from build123d import *

# Parameters (mm, degrees)
BOSS_EXTRUDE1_DEPTH     = 8
SKETCH1_W               = 122.5
SKETCH1_H               = 80
BOSS_EXTRUDE1_2_DEPTH   = 8
BOSS_EXTRUDE2_DEPTH     = 53.5
CUT_EXTRUDE6_DEPTH      = 7.5
SKETCH2_W               = 60
SKETCH2_H               = 31
SKETCH2_R               = 2.25
BOSS_EXTRUDE3_DEPTH     = 31.5
CUT_EXTRUDE5_REACH      = 165.406
SKETCH8_W               = 15.75
SKETCH8_H               = 31
CUT_EXTRUDE8_START      = -3
CUT_EXTRUDE8_DEPTH      = 3
FILLET1_R               = 3
CUT_EXTRUDE1_DEPTH      = 122.5
CUT_EXTRUDE1_DEPTH_BACK = 15
SKETCH4_W               = 3
SKETCH4_H               = 87.5
BOSS_EXTRUDE5_DEPTH     = 122.5
SKETCH5_W               = 5
SKETCH5_H               = 80
CUT_EXTRUDE2_DEPTH      = 122.5
CUT_EXTRUDE3_DEPTH      = 15
CUT_EXTRUDE3_DEPTH_BACK = 92.5
SKETCH7_R               = 2.25
CUT_EXTRUDE4_DEPTH      = 13.5
CUT_EXTRUDE9_DEPTH      = 5
SKETCH13_R              = 1.75
CUT_EXTRUDE10_DEPTH     = 7.5


with BuildPart() as part:
    # Sketch1 → Boss-Extrude1 (new body)
    with BuildSketch(Plane.XY):
        Polygon((32.428932188, 92.5), (27.5, 92.5), (27.5, 7.5), (-92.5, 7.5), (-92.5, -92.5), (92.5, -92.5), (92.5, 32.428932188), align=None)
    extrude(amount=BOSS_EXTRUDE1_DEPTH)



with BuildPart() as body_2:
    # Sketch1 → Boss-Extrude1 2 (new body)
    with BuildSketch(Plane.XY):
        with Locations((-38.75, 52.5)):
            Rectangle(SKETCH1_W, SKETCH1_H)
    extrude(amount=BOSS_EXTRUDE1_2_DEPTH)


with BuildPart() as part_1:
    add(part.part)

    add(body_2.part)  # Boss-Extrude2 merges body 2
    # Sketch1<4> → Boss-Extrude2 (add)
    with BuildSketch(Plane.XY):
        Polygon((22.5, 92.5), (22.5, 12.5), (-100, 12.5), (-100, -100), (100, -100), (100, 32), (32, 100), (-100, 100), (-100, 92.5), align=None)
        Polygon((-92.5, 7.5), (27.5, 7.5), (27.5, 92.5), (32.428932188, 92.5), (92.5, 32.428932188), (92.5, -92.5), (-92.5, -92.5), align=None, mode=Mode.SUBTRACT)
    extrude(amount=BOSS_EXTRUDE2_DEPTH)

    # Sketch9 → Cut-Extrude6 (cut)
    with BuildSketch(Plane.XZ.offset(100)):
        with BuildLine():
            Line((-90, 42.466293919), (90, 42.466293919))
            ThreePointArc((90, 42.466293919), (94, 46.466293919), (90, 50.466293919))
            Line((90, 50.466293919), (-90, 50.466293919))
            ThreePointArc((-90, 50.466293919), (-94, 46.466293919), (-90, 42.466293919))
        make_face()
        with BuildLine():
            Line((-90, 26.466293919), (90, 26.466293919))
            ThreePointArc((90, 26.466293919), (94, 30.466293919), (90, 34.466293919))
            Line((90, 34.466293919), (-90, 34.466293919))
            ThreePointArc((-90, 34.466293919), (-94, 30.466293919), (-90, 26.466293919))
        make_face()
        with BuildLine():
            Line((-90, 10.466293919), (90, 10.466293919))
            ThreePointArc((90, 10.466293919), (94, 14.466293919), (90, 18.466293919))
            Line((90, 18.466293919), (-90, 18.466293919))
            ThreePointArc((-90, 18.466293919), (-94, 14.466293919), (-90, 10.466293919))
        make_face()
    extrude(amount=-CUT_EXTRUDE6_DEPTH, mode=Mode.SUBTRACT)

    # Sketch2 → Boss-Extrude3 (add)
    with BuildSketch(Plane.XY.offset(8)):
        with Locations((12.359091867, -30)):
            Rectangle(SKETCH2_W, SKETCH2_H)
        with BuildLine():
            ThreePointArc((-14.640908133, -38.997517342), (-11.721838066, -37.877814495), (-10.5, -35))
            Line((-10.5, -35), (-10.5, -25))
            ThreePointArc((-10.5, -25), (-11.721838066, -22.122185505), (-14.640908133, -21.002482658))
            Line((-14.640908133, -21.002482658), (-14.640908133, -17.5))
            Line((-14.640908133, -17.5), (34.640908133, -17.5))
            Line((34.640908133, -17.5), (34.640908133, -21.002482658))
            ThreePointArc((34.640908133, -21.002482658), (31.721838066, -22.122185505), (30.5, -25))
            Line((30.5, -25), (30.5, -35))
            ThreePointArc((30.5, -35), (31.721838066, -37.877814495), (34.640908133, -38.997517342))
            Line((34.640908133, -38.997517342), (34.640908133, -42.5))
            Line((34.640908133, -42.5), (-14.640908133, -42.5))
            Line((-14.640908133, -42.5), (-14.640908133, -38.997517342))
        make_face(mode=Mode.SUBTRACT)
        with Locations((-14.5, -25)):
            Circle(SKETCH2_R, mode=Mode.SUBTRACT)
        with Locations((-14.5, -35)):
            Circle(SKETCH2_R, mode=Mode.SUBTRACT)
        with Locations((34.5, -35)):
            Circle(SKETCH2_R, mode=Mode.SUBTRACT)
        with Locations((34.5, -25)):
            Circle(SKETCH2_R, mode=Mode.SUBTRACT)
    extrude(amount=BOSS_EXTRUDE3_DEPTH)

    # Cut-Extrude5: up to this face of the body (flat: up to its plane)
    cut_extrude5_end = Plane(part_1.part.faces().sort_by_distance((-10.5, -30, 23.75))[0])
    # Sketch8 → Cut-Extrude5 (cut, up to the picked face)
    with BuildSketch(Plane.ZY.offset(17.640908133), mode=Mode.PRIVATE) as cut_extrude5_sk1:
        with Locations((15.875, -30)):
            Rectangle(SKETCH8_W, SKETCH8_H)
    cut_extrude5_tool1 = split(extrude(cut_extrude5_sk1.sketch, amount=-CUT_EXTRUDE5_REACH, mode=Mode.PRIVATE), bisect_by=cut_extrude5_end, keep=Keep.BOTH, mode=Mode.PRIVATE)
    add(cut_extrude5_tool1.solids().sort_by(Axis((-17.640908, -30, 15.875), (1, 0, 0)))[0], mode=Mode.SUBTRACT)

    # Sketch10 → Cut-Extrude8 (cut)
    with BuildSketch(Plane.XY.offset(8).offset(CUT_EXTRUDE8_START)):
        with BuildLine():
            Line((34.640908133, -42.5), (34.640908133, -38.997517342))
            ThreePointArc((34.640908133, -38.997517342), (31.721838066, -37.877814495), (30.5, -35))
            Line((30.5, -35), (30.5, -25))
            ThreePointArc((30.5, -25), (31.721838066, -22.122185505), (34.640908133, -21.002482658))
            Line((34.640908133, -21.002482658), (34.640908133, -17.5))
            Line((34.640908133, -17.5), (-14.640908133, -17.5))
            Line((-14.640908133, -17.5), (-34.640908133, -17.5))
            Line((-34.640908133, -17.5), (-34.640908133, -42.5))
            Line((-34.640908133, -42.5), (-14.640908133, -42.5))
            Line((-14.640908133, -42.5), (34.640908133, -42.5))
        make_face()
    extrude(amount=CUT_EXTRUDE8_DEPTH, mode=Mode.SUBTRACT)

    # Fillet1
    fillet1_edges = [part_1.edges().sort_by_distance(p)[0] for p in [
        (-10.5, -44, 23.75),
        (-10.5, -16, 23.75),
    ]]
    fillet(fillet1_edges, radius=FILLET1_R)

    # Sketch3 → Cut-Extrude1 (cut, two sides: drawn at the far end of the back side and taken through both)
    with BuildSketch(Plane.ZY.offset(-22.5).offset(-CUT_EXTRUDE1_DEPTH_BACK)):
        with BuildLine():
            Line((14, 72.5), (14, 32.5))
            ThreePointArc((14, 32.5), (10, 28.5), (6, 32.5))
            Line((6, 32.5), (6, 72.5))
            ThreePointArc((6, 72.5), (10, 76.5), (14, 72.5))
        make_face()
        with BuildLine():
            Line((40.75, 72.5), (40.75, 32.5))
            ThreePointArc((40.75, 32.5), (36.75, 28.5), (32.75, 32.5))
            Line((32.75, 32.5), (32.75, 72.5))
            ThreePointArc((32.75, 72.5), (36.75, 76.5), (40.75, 72.5))
        make_face()
    extrude(amount=CUT_EXTRUDE1_DEPTH + CUT_EXTRUDE1_DEPTH_BACK, mode=Mode.SUBTRACT)

    # Sketch4 → Boss-Extrude5 (add)
    with BuildSketch(Plane.ZY.offset(-22.5)):
        with Locations((26.75, 56.25)):
            Rectangle(SKETCH4_W, SKETCH4_H)
    extrude(amount=BOSS_EXTRUDE5_DEPTH)

    # Sketch5 → Cut-Extrude2 (cut)
    with BuildSketch(Plane.ZY.offset(100)):
        with Locations((5.5, 52.5)):
            Rectangle(SKETCH5_W, SKETCH5_H)
    extrude(amount=-CUT_EXTRUDE2_DEPTH, mode=Mode.SUBTRACT)

    # Sketch6 → Cut-Extrude3 (cut, two sides: drawn at the far end of the back side and taken through both)
    with BuildSketch(Plane.XZ.offset(-7.5).offset(-CUT_EXTRUDE3_DEPTH_BACK)):
        with BuildLine():
            Line((-78.75, 31.25), (1.25, 31.25))
            ThreePointArc((1.25, 31.25), (8.455515357, 38.455515357), (1.25, 45.661030714))
            Line((1.25, 45.661030714), (-78.75, 45.661030714))
            ThreePointArc((-78.75, 45.661030714), (-85.955515357, 38.455515357), (-78.75, 31.25))
        make_face()
        with BuildLine():
            Line((-82.75, 8), (5.25, 8))
            ThreePointArc((5.25, 8), (5.722135955, 13.236067977), (1.25, 16))
            Line((1.25, 16), (-78.75, 16))
            ThreePointArc((-78.75, 16), (-83.222135955, 13.236067977), (-82.75, 8))
        make_face()
        with BuildLine():
            ThreePointArc((1.25, 6), (3.486067977, 6.527864045), (5.25, 8))
            Line((5.25, 8), (-82.75, 8))
            ThreePointArc((-82.75, 8), (-80.986067977, 6.527864045), (-78.75, 6))
            Line((-78.75, 6), (1.25, 6))
        make_face()
    extrude(amount=CUT_EXTRUDE3_DEPTH + CUT_EXTRUDE3_DEPTH_BACK, mode=Mode.SUBTRACT)

    # Sketch7 → Cut-Extrude4 (cut)
    with BuildSketch(Plane.XY.offset(53.5)):
        with Locations((-96.15, 96.15)):
            Circle(SKETCH7_R)
        with Locations((96.15, 96.15)):
            Circle(SKETCH7_R)
        with Locations((-96.15, -96.15)):
            Circle(SKETCH7_R)
        with Locations((96.15, -96.15)):
            Circle(SKETCH7_R)
    extrude(amount=-CUT_EXTRUDE4_DEPTH, mode=Mode.SUBTRACT)

    # Sketch11 → Cut-Extrude9 (cut)
    with BuildSketch(Plane(origin=(66, 66, 0), x_dir=(0, 0, -1), z_dir=(0.7071067811865488, 0.7071067811865462, 0))):
        with BuildLine():
            ThreePointArc((-25, -20), (-25.512563133, -18.762563133), (-26.75, -18.25))
            Line((-26.75, -18.25), (-26.75, -21.75))
            ThreePointArc((-26.75, -21.75), (-25.512563133, -21.237436867), (-25, -20))
        make_face()
        with BuildLine():
            Line((-26.75, -21.75), (-26.75, -18.25))
            ThreePointArc((-26.75, -18.25), (-28.5, -20), (-26.75, -21.75))
        make_face()
        with BuildLine():
            ThreePointArc((-25, 20), (-25.512563133, 21.237436867), (-26.75, 21.75))
            Line((-26.75, 21.75), (-26.75, 18.25))
            ThreePointArc((-26.75, 18.25), (-25.512563133, 18.762563133), (-25, 20))
        make_face()
        with BuildLine():
            Line((-26.75, 18.25), (-26.75, 21.75))
            ThreePointArc((-26.75, 21.75), (-28.5, 20), (-26.75, 18.25))
        make_face()
    extrude(amount=-CUT_EXTRUDE9_DEPTH, mode=Mode.SUBTRACT)

    # Sketch13 → Cut-Extrude10 (cut)
    with BuildSketch(Plane(origin=(100, 0, 0), x_dir=(0, 0, -1), z_dir=(1, 0, 0))):
        with Locations((-26.75, 10)):
            Circle(SKETCH13_R)
    extrude(amount=-CUT_EXTRUDE10_DEPTH, mode=Mode.SUBTRACT)


solid = part_1.part
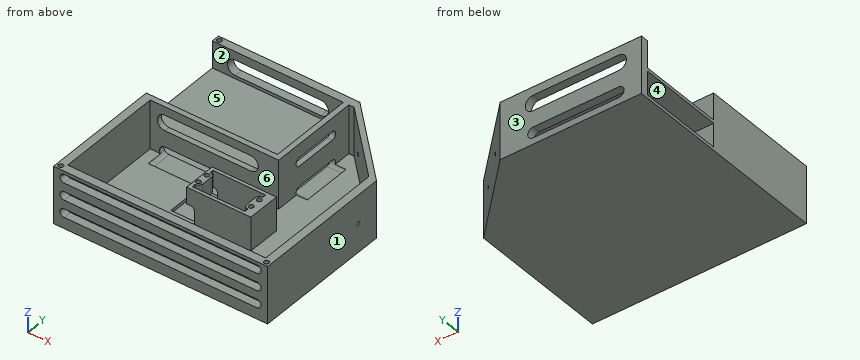
Model file for the job. Use its own axes, mm. Face numbers are marked on the shaded views. A direction names the side the tool comes from. Give positions to 0.01 mm unless a question says otherwise; leave off trailing zeros. Order: outer loops, then holes, each group sorted by start corner. A loop starts at its lowest first (then second) coordinate and runs counter-clockwise, first axis right, second up. Notation, with made-up numbers: (81, 20) - (115, 20) arc R29 ccw to (115, 47) - close; hole circle Ø5 at (-0.75, 76). An arc over 180 degrees is marked (long way). One line per item, written item: value.
Item 1: Two-plate mould, pull along Y, no slides. Class the marked faces 1, 2 and 3: released by +Y, released by -Y, zero draft, split by the parting line, or undercut.
Response values:
face 1: zero draft
face 2: undercut
face 3: released by +Y
Item 2: Pin check, flat tips, straight feed: pin 1 Ø24 at (x, y) = (-34, 48.5) entering from +Z; pin 2 Ø2.5 at (x, y) = (-14.5, -35) entering from +Z; pin 3 Ø6 at (x, y) = (-28.5, 1.5) entering from +Z. Stop position of each tip, or through.
Response values:
pin 1: z = 28.25
pin 2: z = 5
pin 3: z = 6
Item 3: Slice it at B-B (y = 40.5). List the corners of the cut face in (x, z), then the cut area to 3 significant figures.
Response values:
outline: (-100, 0) - (91.5, 0) - (91.5, 53.5) - (84.43, 53.5) - (84.43, 8) - (37.5, 8) - (37.5, 6) - (22.5, 6) - (22.5, 3) - (-100, 3) - close; (-100, 25.25) - (22.5, 25.25) - (22.5, 14) - (27.5, 14) - (27.5, 32.75) - (22.5, 32.75) - (22.5, 28.25) - (-100, 28.25) - close; (22.5, 40.75) - (27.5, 40.75) - (27.5, 53.5) - (22.5, 53.5) - close
area: 1,740 mm2
Item 4: Wall check: line 1 (Y direction, x = -14, z = 34); line 2 (Y direction, x = -96.15, z = 47.25); line 3 (Y direction, x = -2, z = 19.5). Give the ranges that are in metal, low to high.
Response values:
line 1: -45.5 to -42.5, -38.97 to -37.19, -32.81 to -27.19, -22.81 to -21.03, -17.5 to -14.5
line 2: -100 to -98.4, -93.9 to 12.5, 92.5 to 93.9, 98.4 to 100
line 3: -100 to -92.5, -45.5 to -42.5, -17.5 to -14.5, 7.5 to 12.5, 92.5 to 100
Item 5: Slice it at A-A (x = -3). Give the number of separate pieces and of enclosed holes in the cut face, then the cut area to 3 significant figures.
Response values:
separate pieces: 7
enclosed holes: 0
area: 1,950 mm2
Item 6: Tool access for the marked faces 4, 5 and 6: list every direction of +Z, -Z, +X, -X, +Y, -Y with a clear straight run to the whole face (end or side of a thin tool).
Response values:
face 4: -X
face 5: +Z, -X
face 6: +Z
